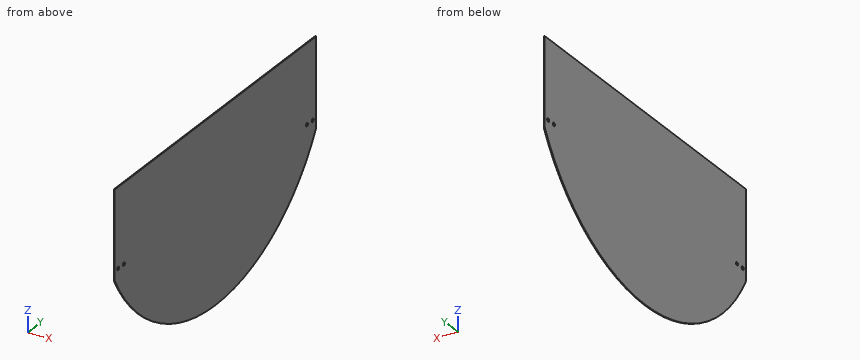
from build123d import *

# Parameters (mm, degrees)
BOSS_EXTRUDE1_DEPTH     = 2.5
SKETCH2_R               = 4.5
CUT_EXTRUDE1_DEPTH      = 10
LPATTERN1_COUNT         = 2
LPATTERN1_PITCH         = 25
MIRROR1_COPY_1_SKETCH_R = 4.5
MIRROR1_COPY_1_DEPTH    = 10


with BuildPart() as part:
    # Sketch1 → Boss-Extrude1 (new body)
    with BuildSketch(Plane(origin=(0, 0, 0), x_dir=(0, 0, -1), z_dir=(1, 0, 0))):
        with BuildLine():
            Line((0, 438), (236.981011898, 438))
            ThreePointArc((236.981011898, 438), (498, 0), (236.981011898, -438))
            Line((236.981011898, -438), (0, -438))
            Line((0, -438), (0, 438))
        make_face()
    extrude(amount=BOSS_EXTRUDE1_DEPTH)

    # Sketch2 → Cut-Extrude1 (cut)
    with BuildSketch(Plane(origin=(2.5, 0, 0), x_dir=(0, 0, -1), z_dir=(1, 0, 0))):
        with Locations((211, 423)):
            Circle(SKETCH2_R)
    cut_extrude1 = extrude(amount=-CUT_EXTRUDE1_DEPTH, mode=Mode.SUBTRACT)

    # LPattern1: Cut-Extrude1 ×2
    with Locations(*[(0, -i * LPATTERN1_PITCH, 0) for i in range(1, LPATTERN1_COUNT)]):
        add(cut_extrude1, mode=Mode.SUBTRACT)

    # Mirror1: Cut-Extrude1 across plane
    add(cut_extrude1.mirror(Plane.ZX), mode=Mode.SUBTRACT)

    # Mirror1 copy 1 sketch → Mirror1 copy 1 (cut)
    with BuildSketch(Plane(origin=(2.5, 25, 0), x_dir=(0, 0, -1), z_dir=(1, 0, 0))):
        with Locations((211, -423)):
            Circle(MIRROR1_COPY_1_SKETCH_R)
    extrude(amount=-MIRROR1_COPY_1_DEPTH, mode=Mode.SUBTRACT)


solid = part.part
Design review of the part built by this model. Coordinates are the model's own, in mm. Round coordinates to 2 decimals unless told otherwise and drop trailing zeros. Write each loop counter-clockwise with the first axis right and the second up, starting at its lowest first coordinate (ties: lowest second). Pieces come first, ordered by that corner, then holes. Notation, with made-up numbers: (-18.75, 6.5) - (22.25, 6.5) arc R20 cw to (22.25, 17.5) - close; hole circle Ø5 at (62, 16). An arc over 180 degrees is marked (long way). Use a Markdown table: item, result. Add a question column.
1. We need section B-B (z = -259). State the section outline as (x, y) points.
2. We need section A-A (x = 1.75). State the section outline as (y, z) points, then the cut area to 3 significant figures.
3. Clearance check with flat-ended pins moving along their axes: pin 1 (1 mm diameter, centred on x = 1.5, z = -347.5, fed in from +Y); pin 2 (1 mm diameter, centred on x = 1.5, z = -389.5, fed in from +Y); pin 3 (5.5 mm diameter, centred on y = 423, z = -211, fed in from -X). State where each tip first meets the part, or that it passes through.
4. We need section C-C (y = -161). State the section outline as (x, z) points.
5. Wall thickness on probe 1 along Y at (x, z) = (1, -211); probe 2 along Z at (x, y) = (1.1, 398); probe 3 along Z at (x, y) = (2.15, 376): over which ranges is each line inside the solid? List them lowest first.
Output:
| question | item | result |
|---|---|---|
| 1 | outline | (0, -425.35) - (2.5, -425.35) - (2.5, 425.35) - (0, 425.35) - close |
| 2 | outline | (-438, -236.98) arc R498 ccw to (438, -236.98) - (438, 0) - (-438, 0) - close; hole circle Ø9 at (-423, -211); hole circle Ø9 at (-398, -211); hole circle Ø9 at (398, -211); hole circle Ø9 at (423, -211) |
| 2 | area | 370,000 mm2 |
| 3 | pin 1 | stops at y = 357.2 |
| 3 | pin 2 | stops at y = 310.94 |
| 3 | pin 3 | passes through |
| 4 | outline | (0, -471.26) - (2.5, -471.26) - (2.5, 0) - (0, 0) - close |
| 5 | probe 1 | y = -438 to -427.5, -418.5 to -402.5, -393.5 to 393.5, 402.5 to 418.5, 427.5 to 438 |
| 5 | probe 2 | z = -299.33 to -215.5, -206.5 to 0 |
| 5 | probe 3 | z = -326.54 to 0 |
